Verification items for the finished model (mm, model axes). Round coordinates to 2 decimals unless told otherwise and drop trailing zeros. Write each loop counter-clockwise with the first axis right and the second up, starting at its lowest first coordinate (ties: lowest second). Pieces come first, ordered by that corner, then holes. Notation, with made-up numbers: (40.25, -18.5) -> (81.25, -18.5) arc R25 cw to (81.25, 11.5) -> close; hole circle Ø2 at (-22.75, 66.25). An arc over 180 degrees is marked (long way). Use CSV: the item, a comma, the result in double quotes.
Autodesk Inventor part; units mm, degrees
ref_plane "YZ Plane" through (0, 0, 0) normal (1, 0, 0) x (0, 1, 0)
ref_plane "XZ Plane" through (0, 0, 0) normal (0, 1, 0) x (-1, 0, 0)
ref_plane "XY Plane" through (0, 0, 0) normal (0, 0, 1) x (1, 0, 0)
sketch "Skizze1" plane through (0, 0, 0) normal (0, 0, 1) x (1, 0, 0)
  line L0 (0, 53.34) -> (0, 0)
  line L1 (0, 0) -> (49.53, 0)
  line L2 (49.53, 0) -> (49.53, 2.54)
  line L3 (49.53, 2.54) -> (52.07, 5.08)
  line L4 (52.07, 5.08) -> (52.07, 38.1)
  line L5 (52.07, 38.1) -> (49.53, 40.64)
  line L6 (49.53, 40.64) -> (49.53, 52.07)
  line L7 (49.53, 52.07) -> (48.26, 53.34)
  line L8 (48.26, 53.34) -> (0, 53.34)
  circle A0 centre (34.29, 38.81) radius 0.45
  circle A1 centre (34.29, 32.31) radius 0.45
  circle A2 centre (46.99, 50.8) radius 0.51
  circle A3 centre (44.45, 50.8) radius 0.51
  circle A4 centre (41.91, 50.8) radius 0.51
  circle A5 centre (39.37, 50.8) radius 0.51
  circle A6 centre (36.83, 50.8) radius 0.51
  circle A7 centre (34.29, 50.8) radius 0.51
  circle A8 centre (31.75, 50.8) radius 0.51
  circle A9 centre (29.21, 50.8) radius 0.51
  circle A10 centre (34.29, 2.54) radius 0.51
  circle A11 centre (36.83, 2.54) radius 0.51
  circle A12 centre (39.37, 2.54) radius 0.51
  circle A13 centre (41.91, 2.54) radius 0.51
  circle A14 centre (44.45, 2.54) radius 0.51
  circle A15 centre (46.99, 2.54) radius 0.51
  circle A16 centre (25.02, 50.8) radius 0.51
  circle A17 centre (22.48, 50.8) radius 0.51
  circle A18 centre (19.94, 50.8) radius 0.51
  circle A19 centre (17.4, 50.8) radius 0.51
  circle A20 centre (14.86, 50.8) radius 0.51
  circle A21 centre (12.32, 50.8) radius 0.51
  circle A22 centre (9.78, 50.8) radius 0.51
  circle A23 centre (7.24, 50.8) radius 0.51
  circle A24 centre (16.51, 2.54) radius 0.51
  circle A25 centre (19.05, 2.54) radius 0.51
  circle A26 centre (21.59, 2.54) radius 0.51
  circle A27 centre (24.13, 2.54) radius 0.51
  circle A28 centre (26.67, 2.54) radius 0.51
  circle A29 centre (29.21, 2.54) radius 0.51
  circle A30 centre (46.99, 30.48) radius 0.51
  circle A31 centre (49.53, 30.48) radius 0.51
  circle A32 centre (46.99, 27.94) radius 0.51
  circle A33 centre (49.53, 27.94) radius 0.51
  circle A34 centre (46.99, 25.4) radius 0.51
  circle A35 centre (49.53, 25.4) radius 0.51
  circle A36 centre (4.65, 13.08) radius 1.5
  circle A37 centre (7.65, 8.38) radius 1.5
  circle A38 centre (10.65, 13.08) radius 1.5
  circle A39 centre (13.97, 36.83) radius 0.51
  circle A40 centre (13.97, 39.37) radius 0.51
  circle A41 centre (1.27, 11.43) radius 0.51
  circle A42 centre (1.27, 13.97) radius 0.51
  circle A43 centre (8.255, 30.48) radius 0.7
  circle A44 centre (8.255, 20.32) radius 0.7
  circle A45 centre (11.66, 1.778) radius 0.45
  circle A46 centre (8.66, 1.778) radius 0.45
  circle A47 centre (2.54, 50.8) radius 1.651
  circle A48 centre (2.54, 2.54) radius 1.651
  circle A49 centre (49.53, 35.56) radius 1.651
  circle A50 centre (49.53, 7.62) radius 1.651
  circle A51 centre (37.719, 14.986) radius 0.254
  circle A52 centre (29.845, 22.86) radius 0.254
  circle A53 centre (22.225, 22.86) radius 0.254
  circle A54 centre (44.831, 16.51) radius 0.254
  circle A55 centre (13.97, 8.89) radius 0.254
  circle A56 centre (35.56, 17.78) radius 0.254
  circle A57 centre (34.671, 18.923) radius 0.254
  circle A58 centre (9.398, 5.08) radius 0.254
  circle A59 centre (39.37, 16.891) radius 0.254
  circle A60 centre (31.75, 2.54) radius 0.254
  circle A61 centre (15.24, 34.29) radius 0.254
  circle A62 centre (20.32, 26.67) radius 0.254
  circle A63 centre (43.307, 30.607) radius 0.254
  circle A64 centre (36.322, 16.51) radius 0.254
  circle A65 centre (20.32, 29.21) radius 0.254
  circle A66 centre (43.18, 33.02) radius 0.254
  circle A67 centre (38.0746, 16.51) radius 0.254
  circle A68 centre (50.8, 16.51) radius 0.254
  circle A69 centre (19.05, 11.43) radius 0.254
extrude "Arduino-Pro-v14.brd_Kontur" add sketch "Skizze1" along normal blind 1.6
properties part number "Arduino-Pro-v14.brd_Kontur"
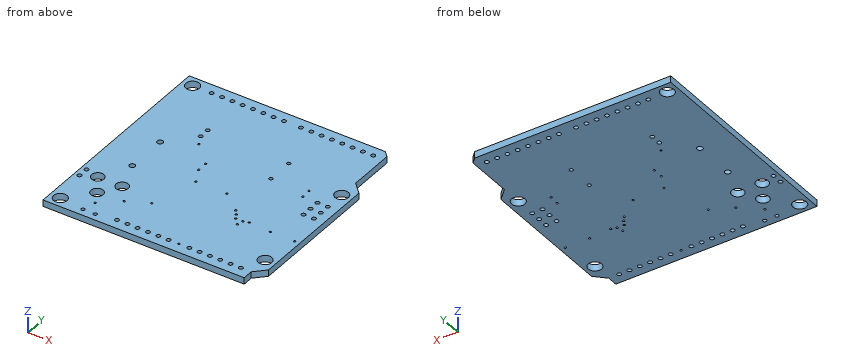
Q1. Section check B-B (y = 47). Record the cut outline in (x, z).
Filled in:
outline,"(0, 0) -> (49.53, 0) -> (49.53, 1.6) -> (0, 1.6) -> close"
Q2. Section check A-A (z = 0.4). State how many separate pieces and enclosed holes the cut face has, plus the area to 3 significant figures.
Filled in:
separate pieces,"1"
enclosed holes,"70"
area,"2,640 mm²"
Q3. Material ranges on L1, parallel to Y at x = 14, z = 0.4; L2, parallel to Y at x = 39.37, z = 1.2 (3 decimals); L3, parallel to X at y = 29.21, z = 0.35, recorded low to high.
Filled in:
L1,"0 to 8.64, 9.14 to 36.32, 37.34 to 38.86, 39.88 to 53.34"
L2,"0 to 2.03, 3.05 to 16.637, 17.145 to 50.29, 51.31 to 53.34"
L3,"0 to 20.07, 20.57 to 52.07"
